Autodesk Inventor part; units mm, degrees
ref_plane "YZ Plane" through (0, 0, 0) normal (1, 0, 0) x (0, 1, 0)
ref_plane "XZ Plane" through (0, 0, 0) normal (0, 1, 0) x (-1, 0, 0)
ref_plane "XY Plane" through (0, 0, 0) normal (0, 0, 1) x (1, 0, 0)
sketch "Sketch1" plane through (0, 0, 0) normal (0, 0, 1) x (1, 0, 0)
  circle A0 centre (0, 0) radius 15
  dimension "d0" = 30
extrude "Extrusion1" add sketch "Sketch1" along normal blind 3
sketch "Sketch2" plane through (0, 0, 3) normal (0, 0, 1) x (1, 0, 0)
  circle A0 centre (0, 0) radius 15
  circle A1 centre (0, 0) radius 12.5
  dimension "d4" = 25
extrude "Extrusion2" add sketch "Sketch2" along normal blind 4 contours A1
sketch "Sketch3" plane through (0, 0, 7) normal (0, 0, 1) x (1, 0, 0)
  circle A0 centre (0, 0) radius 12.5
  circle A1 centre (0, 0) radius 15
extrude "Extrusion3" add sketch "Sketch3" along normal blind 3 contours A0 | A1
fillet "Fillet1" radius 2 4 edges at (-15, 0, 3) (-12.5, 0, 3) (-15, 0, 7) (-12.5, 0, 7)
sketch "Sketch5" plane through (0, 0, 0) normal (0, 0, -1) x (-1, 0, 0)
  circle A0 centre (0, 0) radius 15
  circle A1 centre (0, 0) radius 3.5
  dimension "d15" = 7
extrude "Extrusion5" cut sketch "Sketch5" against normal blind 4 contours A1
sketch "Sketch6" plane through (0, 0, 4) normal (0, 0, -1) x (-1, 0, 0)
  circle A0 centre (0, 0) radius 3.5
  circle A1 centre (0, 0) radius 3.6
  dimension "d19" = 7.2
extrude "Extrusion6" cut sketch "Sketch6" against normal blind 4 contours A0 | A1
sketch "Sketch7" plane through (0, 0, 10) normal (0, 0, 1) x (1, 0, 0)
  circle A0 centre (0, 0) radius 15
  circle A1 centre (0, 0) radius 8
  dimension "d24" = 16
extrude "Extrusion7" cut sketch "Sketch7" against normal blind 8 contours A1
sketch "Sketch8" plane through (0, 0, 2) normal (0, 0, 1) x (1, 0, 0)
  circle A0 centre (0, 0) radius 8
  circle A1 centre (0, 0) radius 6
  circle A2 centre (0, 0) radius 4
  dimension "d28" = 12
  dimension "d30" = 8
extrude "Extrusion8" add sketch "Sketch8" along normal blind 3.8 contours A1
properties part number "Wire guidance wheelV2"
Check sheet for the modelled part. Datum: model origin and axes. Units: mm. A direction names the side the tool comes from. Round coordinates to 2 decimals unless told otherwise and drop trailing zeros. Write each loop counter-clockwise with the first axis right and the second up, starting at its lowest first coordinate (ties: lowest second). Pieces come first, ordered by that corner, then holes. Notation, with made-up numbers: (3, 86) -> (20, 86) arc R21 cw to (20, 115) -> close; hole circle Ø6 at (57.5, 1.5). An arc over 180 degrees is marked (long way). Answer as CSV lines item,"result". Start each with the question number.
1) Material ranges on line 1 (Y direction, x = 0, z = 0.95); line 2 (Y direction, x = 0, z = 3.3); line 3 (Y direction, x = 0, z = 6), recorded low to high. Write a range as from..to.
2) Tool access check on faces 5 (the cylindrical face through (-6, 0, 4)), 6 (the cylindrical face through (-14.985, -0.66, 0.493)). Record the directions out of +Z, -Z, +X, -X, +Y, -Y that give a thin tool (end or side, any length) a straight path to the whole face; none if there is none.
3) Go/stop test with flat-tipped pins: P1, Ø6, axis at x = -6.5, z = 1, coming from the -Y side; P2, Ø3, axis at y = 7.5, z = 8.5, coming from the -X side; P3, Ø17.5, axis at x = -4, y = 2.5, coming from the +Z side; P4, Ø6, axis at x = 2, y = 1.5, coming from the +Z side. Record where each tip stops, or that it passes through.
4) Section check B-B on z = 3.5. State how many separate pieces and enclosed holes the cut face has, and give its area (3 significant figures).
5) Section check A-A on z = 7.75. Enter the section's corners in (x, y).
6) Release check for a two-part mould opening along Y. For faces 1 (the flat face through (-2, 6, 2)), 2 (the cylindrical face through (-9.92, 7.606, 4.996)), 3 (the cylindrical face through (-0.867, 3.905, 3.873)), 4 (the flat face through (6, -6, 10)) record: pulls with the +Y half, pulls with the -Y half, needs draft (parallel to the pull), parting line crosses it, or undercut.
Found:
1,line 1,"y = -15..-3.5, 3.5..15"
1,line 2,"y = -13.08..-8, -6..-4, 4..6, 8..13.08"
1,line 3,"y = -12.63..-8, 8..12.63"
2,face 5,"+Z"
2,face 6,"+Z, -Z"
3,P1,"stops at y = -14.59"
3,P2,"stops at x = -13.72"
3,P3,"stops at z = 10"
3,P4,"stops at z = 5.8"
4,separate pieces,"2"
4,enclosed holes,"2"
4,area,"385 mm^2"
5,outline,"circle Ø29.12 at (0, 0); hole circle Ø16 at (0, 0)"
6,face 1,"undercut"
6,face 2,"parting line crosses it"
6,face 3,"undercut"
6,face 4,"needs draft"
